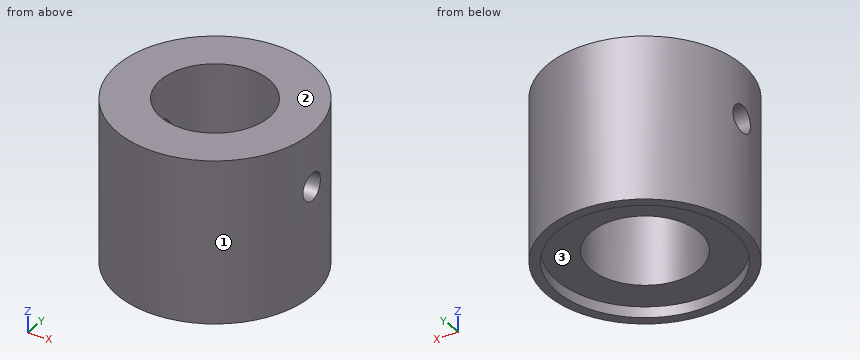
from build123d import *

# Parameters (mm, degrees)
ESQUISSE1_R             = 9
ESQUISSE1_R_2           = 5
BOSS_EXTRU_1_DEPTH      = 15
TROU_TARAUD_M31_D       = 2.5
TROU_TARAUD_M31_DEPTH   = 8.5
TROU_TARAUD_M31_TIP     = 0.751075774
TROU_TARAUD_M32_D       = 2.5
TROU_TARAUD_M32_DEPTH   = 8.5
TROU_TARAUD_M32_TIP     = 0.751075774
ESQUISSE9_R             = 8.1
ENL_V_MAT_EXTRU_1_DEPTH = 1


with BuildPart() as part:
    # Esquisse1 → Boss.-Extru.1 (new body)
    with BuildSketch(Plane.XY):
        Circle(ESQUISSE1_R)
        Circle(ESQUISSE1_R_2, mode=Mode.SUBTRACT)
    extrude(amount=BOSS_EXTRU_1_DEPTH)

    # Trou taraudé M31
    with Locations(Plane(origin=(9, 0, 0), x_dir=(0, 0, -1), z_dir=(1, 0, 0))):
        with Locations((-10, 0)):
            Hole(TROU_TARAUD_M31_D / 2, depth=TROU_TARAUD_M31_DEPTH)
            with Locations((0, 0, -(TROU_TARAUD_M31_DEPTH + TROU_TARAUD_M31_TIP / 2))):  # 118° drill point
                Cone(0, TROU_TARAUD_M31_D / 2, TROU_TARAUD_M31_TIP, mode=Mode.SUBTRACT)

    # Trou taraudé M32
    with Locations(Plane(origin=(-9, 0, 0), x_dir=(0, 0, -1), z_dir=(-1, 0, 0))):
        with Locations((-10, 0)):
            Hole(TROU_TARAUD_M32_D / 2, depth=TROU_TARAUD_M32_DEPTH)
            with Locations((0, 0, -(TROU_TARAUD_M32_DEPTH + TROU_TARAUD_M32_TIP / 2))):  # 118° drill point
                Cone(0, TROU_TARAUD_M32_D / 2, TROU_TARAUD_M32_TIP, mode=Mode.SUBTRACT)

    # Esquisse9 → Enlèv. mat.-Extru.1 (cut)
    with BuildSketch(Plane(origin=(0, 0, 0), x_dir=(-1, 0, 0), z_dir=(0, 0, -1))):
        Circle(ESQUISSE9_R)
    extrude(amount=-ENL_V_MAT_EXTRU_1_DEPTH, mode=Mode.SUBTRACT)


solid = part.part
Verification items for the finished model (mm, model axes). Face numbers are marked on the shaded views. Coordinates: 2 decimals unless noted, no trailing zeros. Order: outer loops, then holes, each group sorted by start corner. A loop starts at its lowest first (then second) coordinate and runs counter-clockwise, first axis right, second up. Notation, with made-up numbers: (34, 48.5) -> (78, 48.5) arc R25 cw to (78, 65.5) -> close; hole circle Ø6 at (8, -35). An arc over 180 degrees is marked (long way). Put each result on its own line as item: value. Start each with the question number.
1. Cross-section at A-A, the plane y = 0. Record the boundary of the cut face in (x, z), then the cut area to 3 significant figures.
2. Cross-section at C-C, the plane z = 9. Record the boundary of the cut face in (x, y).
3. Go/stop test with flat-tipped pins: pin 1 Ø6 at (y, z) = (-7, 3.5) entering from -X; pin 2 Ø1.5 at (x, z) = (-1, 7.5) entering from -Y; pin 3 Ø2 at (y, z) = (0, 10) entering from +X; pin 4 Ø1 at (y, z) = (5.5, 10) entering from +X. Record where each tip stops, or that it passes through.
4. Cross-section at D-D, the plane x = -5.5. Record the boundary of the cut face in (y, z).
5. Cross-section at B-B, the plane x = 0. Record the boundary of the cut face in (y, z), then the cut area to 3 significant figures.
6. Mould release check, pull along Y, two halves, no side actions. Record for the marked faces 1, 2 and 3: released by +Y, released by -Y, zero draft, split by the parting line, or undercut.
7. Material ranges on L1, parallel to Y at x = 0, z = 0.35; L2, parallel to Z at x = -2.75, y = 7.5; L3, parallel to Z at x = 5.5, y = 0, recorded low to high. Write a range as [from, to].
Computed:
1. outline: (-9, 0) -> (-8.1, 0) -> (-8.1, 1) -> (-5, 1) -> (-5, 8.75) -> (-9, 8.75) -> close; (-9, 11.25) -> (-5, 11.25) -> (-5, 15) -> (-9, 15) -> close; (5, 1) -> (8.1, 1) -> (8.1, 0) -> (9, 0) -> (9, 8.75) -> (5, 8.75) -> close; (5, 11.25) -> (9, 11.25) -> (9, 15) -> (5, 15) -> close
1. area: 93.8 mm2
2. outline: (-8.97, -0.75) arc R9 ccw to (8.97, -0.75) -> (4.94, -0.75) arc R5 cw to (-4.94, -0.75) -> close; (-8.97, 0.75) -> (-4.94, 0.75) arc R5 cw to (4.94, 0.75) -> (8.97, 0.75) arc R9 ccw to start
3. pin 1: x = -8.06
3. pin 2: y = -9
3. pin 3: through
3. pin 4: x = 7.48
4. outline: (-7.12, 0) -> (-5.95, 0) -> (-5.95, 1) -> (5.95, 1) -> (5.95, 0) -> (7.12, 0) -> (7.12, 15) -> (-7.12, 15) -> close; hole circle Ø2.5 at (0, 10)
5. outline: (-9, 0) -> (-8.1, 0) -> (-8.1, 1) -> (-5, 1) -> (-5, 15) -> (-9, 15) -> close; (5, 1) -> (8.1, 1) -> (8.1, 0) -> (9, 0) -> (9, 15) -> (5, 15) -> close
5. area: 114 mm2
6. face 1: split by the parting line
6. face 2: zero draft
6. face 3: undercut
7. L1: [-9, -8.1], [8.1, 9]
7. L2: [1, 15]
7. L3: [1, 8.75], [11.25, 15]
